Model file for the job. Use its own axes, mm. A direction names the side the tool comes from. Give positions to 0.01 mm unless a question says otherwise; leave off trailing zeros. Order: outer loops, then holes, each group sorted by start corner. A loop starts at its lowest first (then second) coordinate and runs counter-clockwise, first axis right, second up. Notation, with made-up numbers: (15.25, -29.75) - (19.25, -29.75) arc R26 cw to (19.25, -6.75) - close; hole circle Ø8 at (8, 61.5). An arc over 180 degrees is marked (long way). Return JSON: item names as keys, results as strings. Group by question number.
from build123d import *

# Parameters (mm, degrees)
IZIM1_R                       = 22.5
IZIM1_R_2                     = 16.1
Y_KSEKLIK_EKSTR_ZYON1_DEPTH   = 8.25
IZIM1_R_3                     = 35.05
IZIM1_R_4                     = 31
Y_KSEKLIK_EKSTR_ZYON1_2_DEPTH = 8.25
IZIM2_R                       = 1.5
IZIM2_R_2                     = 7.15
Y_KSEKLIK_EKSTR_ZYON2_DEPTH   = 5
IZIM7_R                       = 16.1
KES_EKSTR_ZYON2_DEPTH         = 1
IZIM8_R                       = 8.25
KES_EKSTR_ZYON3_DEPTH         = 4
KES_EKSTR_ZYON4_REACH         = 69.776
IZIM9_R                       = 1.45
IZIM10_R                      = 1.5
KES_EKSTR_ZYON5_DEPTH         = 5
IZIM11_R                      = 12.5
KES_EKSTR_ZYON6_DEPTH         = 2


with BuildPart() as part:
    # izim1 → Y_kseklik-Ekstr_zyon1 (new body)
    with BuildSketch(Plane.XY):
        Circle(IZIM1_R)
        Circle(IZIM1_R_2, mode=Mode.SUBTRACT)
    extrude(amount=Y_KSEKLIK_EKSTR_ZYON1_DEPTH)



with BuildPart() as body_2:
    # izim1 → Y_kseklik-Ekstr_zyon1 2 (new body)
    with BuildSketch(Plane.XY):
        Circle(IZIM1_R_3)
        Circle(IZIM1_R_4, mode=Mode.SUBTRACT)
    extrude(amount=Y_KSEKLIK_EKSTR_ZYON1_2_DEPTH)


with BuildPart() as part_1:
    add(part.part)

    add(body_2.part)  # Y_kseklik-Ekstr_zyon2 merges body 2
    # izim2 → Y_kseklik-Ekstr_zyon2 (add)
    with BuildSketch(Plane.XY.offset(8.25)):
        with BuildLine():
            ThreePointArc((-10.540830255, 39.621848739), (-28.991378029, 28.991378029), (-39.621848739, 10.540830255))
            ThreePointArc((-39.621848739, 10.540830255), (-41.396931543, 6.966269622), (-44.428571429, 4.370588155))
            ThreePointArc((-44.428571429, 4.370588155), (-47, 0), (-44.428571429, -4.370588155))
            ThreePointArc((-44.428571429, -4.370588155), (-41.396931543, -6.966269622), (-39.621848739, -10.540830255))
            ThreePointArc((-39.621848739, -10.540830255), (-28.991378029, -28.991378029), (-10.540830255, -39.621848739))
            ThreePointArc((-10.540830255, -39.621848739), (-6.966269622, -41.396931543), (-4.370588155, -44.428571429))
            ThreePointArc((-4.370588155, -44.428571429), (0, -47), (4.370588155, -44.428571429))
            ThreePointArc((4.370588155, -44.428571429), (6.966269622, -41.396931543), (10.540830255, -39.621848739))
            ThreePointArc((10.540830255, -39.621848739), (28.991378029, -28.991378029), (39.621848739, -10.540830255))
            ThreePointArc((39.621848739, -10.540830255), (41.396931543, -6.966269622), (44.428571429, -4.370588155))
            ThreePointArc((44.428571429, -4.370588155), (47, 0), (44.428571429, 4.370588155))
            ThreePointArc((44.428571429, 4.370588155), (41.396931543, 6.966269622), (39.621848739, 10.540830255))
            ThreePointArc((39.621848739, 10.540830255), (28.991378029, 28.991378029), (10.540830255, 39.621848739))
            ThreePointArc((10.540830255, 39.621848739), (6.966269622, 41.396931543), (4.370588155, 44.428571429))
            ThreePointArc((4.370588155, 44.428571429), (0, 47), (-4.370588155, 44.428571429))
            ThreePointArc((-4.370588155, 44.428571429), (-6.966269622, 41.396931543), (-10.540830255, 39.621848739))
        make_face()
        with Locations((0, 42)):
            Circle(IZIM2_R, mode=Mode.SUBTRACT)
        with Locations((42, 0)):
            Circle(IZIM2_R, mode=Mode.SUBTRACT)
        with Locations((0, -42)):
            Circle(IZIM2_R, mode=Mode.SUBTRACT)
        with Locations((-42, 0)):
            Circle(IZIM2_R, mode=Mode.SUBTRACT)
        Circle(IZIM2_R_2, mode=Mode.SUBTRACT)
    extrude(amount=Y_KSEKLIK_EKSTR_ZYON2_DEPTH)

    # izim7 → Kes-Ekstr_zyon2 (cut)
    with BuildSketch(Plane(origin=(0, 0, 8.25), x_dir=(-1, 0, 0), z_dir=(0, 0, -1))):
        Circle(IZIM7_R)
    extrude(amount=-KES_EKSTR_ZYON2_DEPTH, mode=Mode.SUBTRACT)

    # izim8 → Kes-Ekstr_zyon3 (cut)
    with BuildSketch(Plane(origin=(0, 0, 9.25), x_dir=(-1, 0, 0), z_dir=(0, 0, -1))):
        Circle(IZIM8_R)
    extrude(amount=-KES_EKSTR_ZYON3_DEPTH, mode=Mode.SUBTRACT)

    # Kes-Ekstr_zyon4: up to this face of the body (flat: up to its plane)
    kes_ekstr_zyon4_end = Plane(part_1.part.faces().sort_by_distance((-21.863603897, 0, 0))[0])
    # izim9 → Kes-Ekstr_zyon4 (cut, up to the picked face)
    with BuildSketch(Plane.XY.offset(13.25), mode=Mode.PRIVATE) as kes_ekstr_zyon4_sk1:
        with Locations((-19.052558883, 11)):
            Circle(IZIM9_R)
    kes_ekstr_zyon4_tool1 = split(extrude(kes_ekstr_zyon4_sk1.sketch, amount=-KES_EKSTR_ZYON4_REACH, mode=Mode.PRIVATE), bisect_by=kes_ekstr_zyon4_end, keep=Keep.BOTH, mode=Mode.PRIVATE)
    # izim9 → Kes-Ekstr_zyon4 (cut, up to the picked face)
    with BuildSketch(Plane.XY.offset(13.25), mode=Mode.PRIVATE) as kes_ekstr_zyon4_sk2:
        with Locations((19.052558883, -11)):
            Circle(IZIM9_R)
    kes_ekstr_zyon4_tool2 = split(extrude(kes_ekstr_zyon4_sk2.sketch, amount=-KES_EKSTR_ZYON4_REACH, mode=Mode.PRIVATE), bisect_by=kes_ekstr_zyon4_end, keep=Keep.BOTH, mode=Mode.PRIVATE)
    # izim9 → Kes-Ekstr_zyon4 (cut, up to the picked face)
    with BuildSketch(Plane.XY.offset(13.25), mode=Mode.PRIVATE) as kes_ekstr_zyon4_sk3:
        with Locations((19.052558883, 11)):
            Circle(IZIM9_R)
    kes_ekstr_zyon4_tool3 = split(extrude(kes_ekstr_zyon4_sk3.sketch, amount=-KES_EKSTR_ZYON4_REACH, mode=Mode.PRIVATE), bisect_by=kes_ekstr_zyon4_end, keep=Keep.BOTH, mode=Mode.PRIVATE)
    # izim9 → Kes-Ekstr_zyon4 (cut, up to the picked face)
    with BuildSketch(Plane.XY.offset(13.25), mode=Mode.PRIVATE) as kes_ekstr_zyon4_sk4:
        with Locations((-19.052558883, -11)):
            Circle(IZIM9_R)
    kes_ekstr_zyon4_tool4 = split(extrude(kes_ekstr_zyon4_sk4.sketch, amount=-KES_EKSTR_ZYON4_REACH, mode=Mode.PRIVATE), bisect_by=kes_ekstr_zyon4_end, keep=Keep.BOTH, mode=Mode.PRIVATE)
    add(kes_ekstr_zyon4_tool1.solids().sort_by(Axis((-19.052559, 11, 13.25), (0, 0, -1)))[0], mode=Mode.SUBTRACT)
    add(kes_ekstr_zyon4_tool2.solids().sort_by(Axis((19.052559, -11, 13.25), (0, 0, -1)))[0], mode=Mode.SUBTRACT)
    add(kes_ekstr_zyon4_tool3.solids().sort_by(Axis((19.052559, 11, 13.25), (0, 0, -1)))[0], mode=Mode.SUBTRACT)
    add(kes_ekstr_zyon4_tool4.solids().sort_by(Axis((-19.052559, -11, 13.25), (0, 0, -1)))[0], mode=Mode.SUBTRACT)

    # izim10 → Kes-Ekstr_zyon5 (cut)
    with BuildSketch(Plane(origin=(0, 0, 8.25), x_dir=(-1, 0, 0), z_dir=(0, 0, -1))):
        with Locations((0, 27.54309269)):
            Circle(IZIM10_R)
        with Locations((9.443282325, 25.873661779)):
            Circle(IZIM10_R)
        with Locations((-9.42029251, 25.882040955)):
            Circle(IZIM10_R)
        with Locations((9.42029251, -25.882040955)):
            Circle(IZIM10_R)
        with Locations((0, -27.54309269)):
            Circle(IZIM10_R)
        with Locations((-9.443282325, -25.873661779)):
            Circle(IZIM10_R)
    extrude(amount=-KES_EKSTR_ZYON5_DEPTH, mode=Mode.SUBTRACT)

    # izim11 → Kes-Ekstr_zyon6 (cut)
    with BuildSketch(Plane(origin=(0, 0, 9.25), x_dir=(-1, 0, 0), z_dir=(0, 0, -1))):
        Circle(IZIM11_R)
    extrude(amount=-KES_EKSTR_ZYON6_DEPTH, mode=Mode.SUBTRACT)


solid = part_1.part
(1) Drop flat-ended pins along their axis: pin 1 Ø2 at (y, z) = (7, 11) entering from -X; pin 2 Ø3.5 at (x, y) = (0, 42) entering from +Z; pin 3 Ø9.5 at (x, y) = (-5, 1.5) entering from -Z; pin 4 Ø4 at (y, z) = (-33, 3.5) entering from +X. Give the stop position or say it passes through.
(2) Slice it at D-D (y = 20.5). Give the cut face in (x, z), and give its area (3 significant figures).
(3) 3-axis set-ups, long thin cutter, end or side, ignore diameter. For faces 4 (the face through (-35, 4, 8.25)), 5 (the face through (-47, 0, 11)): which of +Z, -Z, +X, -X, +Y, -Y reach the whole face in a straight line?
(4) Slice it at B-B (y = -42). Give the cut face in (x, z).
(5) Pull direction Y, two halves, no side cores. Call faces 1 (the face through (0.3, 22.5, 4.1)), 2 (the face through (41.432, 6.922, 10.715)), 3 (the face through (-4.563, 34.752, 4.067)): released by +Y, released by -Y, zero draft, split by the parting line, or undercut.
(6) Drill centre lines: L1, parallel to Y at x = -1.5, z = 4; L2, parallel to Y at x = 8, z = 4.75; L3, parallel to X at y = -11, z = 4. Where is each one in solid material? Low to high.
(7) Slice it at A-A (z = 4.5). Give the cut face in (x, y), and give its area (3 significant figures).
Result set:
{
 "1": {"pin 1": "stops at x = -42.26", "pin 2": "stops at z = 13.25", "pin 3": "stops at z = 11.25", "pin 4": "stops at x = 16.36"},
 "2": {"outline": "(-35.51, 8.25) - (-28.43, 8.25) - (-28.43, 0) - (-23.25, 0) - (-23.25, 8.25) - (-9.27, 8.25) - (-9.27, 0) - (9.27, 0) - (9.27, 8.25) - (23.25, 8.25) - (23.25, 0) - (28.43, 0) - (28.43, 8.25) - (35.51, 8.25) - (35.51, 13.25) - (-35.51, 13.25) - close", "area": "593 mm²"},
 "3": {"face 4": "-Z", "face 5": "+Z, -Z, -X"},
 "4": {"outline": "(-6.26, 8.25) - (-1.5, 8.25) - (-1.5, 13.25) - (-6.26, 13.25) - close; (1.5, 8.25) - (6.26, 8.25) - (6.26, 13.25) - (1.5, 13.25) - close"},
 "5": {"face 1": "undercut", "face 2": "released by +Y", "face 3": "split by the parting line"},
 "6": {"L1": "y = -35.02 to -30.96, -22.45 to -16.03, 16.03 to 22.45, 30.96 to 35.02", "L2": "y = -34.12 to -29.95, -21.03 to -13.97, 13.97 to 21.03, 29.95 to 34.12", "L3": "x = -33.28 to -28.98, -17.6 to -11.76, 11.76 to 17.6, 28.98 to 33.28"},
 "7": {"outline": "circle Ø70.1 at (0, 0); (-20.14, -10.04) arc R1.45 cw (long way) to (-18.76, -12.42) arc R22.5 ccw to (18.76, -12.42) arc R1.45 cw (long way) to (20.14, -10.04) arc R22.5 ccw to (20.14, 10.04) arc R1.45 cw (long way) to (18.76, 12.42) arc R22.5 ccw to (-18.76, 12.42) arc R1.45 cw (long way) to (-20.14, 10.04) arc R22.5 ccw to start; hole circle Ø62 at (0, 0); hole circle Ø32.2 at (0, 0)", "area": "1,600 mm²"}
}
